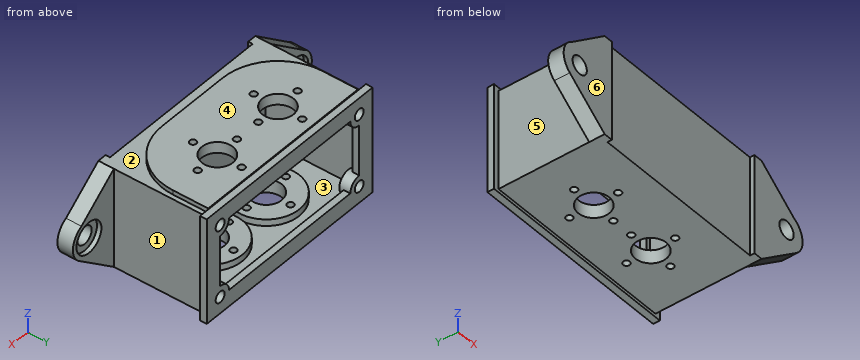
```python
from build123d import *

# Parameters (mm, degrees)
BOSS_EXTRUDE5_DEPTH  = 7
SKETCH10_W           = 88
SKETCH10_H           = 45
SKETCH10_W_2         = 82
SKETCH10_H_2         = 39
BOSS_EXTRUDE6_DEPTH  = 41
SKETCH11_W           = 93
SKETCH11_H           = 48
SKETCH11_W_2         = 78
SKETCH11_H_2         = 33
BOSS_EXTRUDE7_DEPTH  = 3
SKETCH12_R           = 5
BOSS_EXTRUDE8_DEPTH  = 5
SKETCH13_R           = 2.5
CUT_EXTRUDE1_DEPTH   = 5
SKETCH14_R           = 15
BOSS_EXTRUDE9_DEPTH  = 3
SKETCH16_R           = 7
CUT_EXTRUDE2_DEPTH   = 22
SKETCH17_R           = 1.5
CUT_EXTRUDE3_DEPTH   = 22
SKETCH18_W           = 80
SKETCH18_H           = 2
CUT_EXTRUDE4_DEPTH   = 92
BOSS_EXTRUDE11_DEPTH = 2
SKETCH20_R           = 7
CUT_EXTRUDE5_DEPTH   = 14
SKETCH21_R           = 1.5
CUT_EXTRUDE6_DEPTH   = 14
SKETCH22_R           = 4
CUT_EXTRUDE8_DEPTH   = 14
SKETCH23_R           = 7
CUT_EXTRUDE9_DEPTH   = 2


with BuildPart() as part:
    # Sketch9 → Boss-Extrude5 (new body)
    with BuildSketch(Plane(origin=(0, 0, 0), x_dir=(1, 0, 0), z_dir=(0, 1, 0))):
        with BuildLine():
            Line((-44, 22.5), (44, 22.5))
            Line((44, 22.5), (63.572502172, 7.067334685))
            ThreePointArc((63.572502172, 7.067334685), (66.961735718, -0.829031319), (62.181462037, -7.969653395))
            Line((62.181462037, -7.969653395), (44, -22.5))
            Line((44, -22.5), (-44, -22.5))
            Line((-44, -22.5), (-62.181462037, -7.969653395))
            ThreePointArc((-62.181462037, -7.969653395), (-66.961735718, -0.829031319), (-63.572502172, 7.067334685))
            Line((-63.572502172, 7.067334685), (-44, 22.5))
        make_face()
    extrude(amount=BOSS_EXTRUDE5_DEPTH)

    # Sketch10 → Boss-Extrude6 (add)
    with BuildSketch(Plane(origin=(0, 7, 0), x_dir=(1, 0, 0), z_dir=(0, 1, 0))):
        Rectangle(SKETCH10_W, SKETCH10_H)
        Rectangle(SKETCH10_W_2, SKETCH10_H_2, mode=Mode.SUBTRACT)
    extrude(amount=BOSS_EXTRUDE6_DEPTH)

    # Sketch11 → Boss-Extrude7 (add)
    with BuildSketch(Plane(origin=(0, 48, 0), x_dir=(1, 0, 0), z_dir=(0, 1, 0))):
        Rectangle(SKETCH11_W, SKETCH11_H)
        Rectangle(SKETCH11_W_2, SKETCH11_H_2, mode=Mode.SUBTRACT)
    extrude(amount=BOSS_EXTRUDE7_DEPTH)

    # Sketch12 → Boss-Extrude8 (add)
    with BuildSketch(Plane(origin=(0, 51, 0), x_dir=(1, 0, 0), z_dir=(0, 1, 0))):
        with Locations((39, 16.5)):
            Circle(SKETCH12_R)
        with Locations((39, -16.5)):
            Circle(SKETCH12_R)
        with Locations((-39, -16.5)):
            Circle(SKETCH12_R)
        with Locations((-39, 16.5)):
            Circle(SKETCH12_R)
    extrude(amount=-BOSS_EXTRUDE8_DEPTH)

    # Sketch13 → Cut-Extrude1 (cut)
    with BuildSketch(Plane(origin=(0, 51, 0), x_dir=(1, 0, 0), z_dir=(0, 1, 0))):
        with Locations(Location((39, 16.5, 0), (0, 0, 270))):
            Circle(SKETCH13_R)
        with Locations(Location((39, -16.5, 0), (0, 0, 323.130102354))):
            Circle(SKETCH13_R)
        with Locations(Location((-39, 16.5, 0), (0, 0, 216.869897646))):
            Circle(SKETCH13_R)
        with Locations(Location((-39, -16.5, 0), (0, 0, 270))):
            Circle(SKETCH13_R)
    extrude(amount=-CUT_EXTRUDE1_DEPTH, mode=Mode.SUBTRACT)

    # Sketch14 → Boss-Extrude9 (add)
    with BuildSketch(Plane.XY.offset(-19.5)):
        with Locations((16, 27.5)):
            Circle(SKETCH14_R)
        with Locations(Location((-16, 27.5, 0), (0, 0, 180))):
            Circle(SKETCH14_R)
    extrude(amount=BOSS_EXTRUDE9_DEPTH)

    # Sketch16 → Cut-Extrude2 (cut)
    with BuildSketch(Plane.XY.offset(-16.5)):
        with Locations((-16, 27.5)):
            Circle(SKETCH16_R)
        with Locations((16, 27.5)):
            Circle(SKETCH16_R)
    extrude(amount=-CUT_EXTRUDE2_DEPTH, mode=Mode.SUBTRACT)

    # Sketch17 → Cut-Extrude3 (cut)
    with BuildSketch(Plane.XY.offset(-16.5)):
        with Locations((16, 38.5)):
            Circle(SKETCH17_R)
        with Locations((27, 27.5)):
            Circle(SKETCH17_R)
        with Locations((16, 16.5)):
            Circle(SKETCH17_R)
        with Locations((5, 27.5)):
            Circle(SKETCH17_R)
        with Locations((-5, 27.5)):
            Circle(SKETCH17_R)
        with Locations((-16, 16.5)):
            Circle(SKETCH17_R)
        with Locations((-27, 27.5)):
            Circle(SKETCH17_R)
        with Locations((-16, 38.5)):
            Circle(SKETCH17_R)
    extrude(amount=-CUT_EXTRUDE3_DEPTH, mode=Mode.SUBTRACT)

    # Sketch18 → Cut-Extrude4 (cut)
    with BuildSketch(Plane.XY.offset(22.5)):
        with Locations((0, 1)):
            Rectangle(SKETCH18_W, SKETCH18_H)
    extrude(amount=-CUT_EXTRUDE4_DEPTH, mode=Mode.SUBTRACT)

    # Sketch19 → Boss-Extrude11 (add)
    with BuildSketch(Plane.XY.offset(22.5)):
        with BuildLine():
            Line((-42, 48), (42, 48))
            Line((42, 48), (42, 32))
            ThreePointArc((42, 32), (34.67766953, 14.32233047), (17, 7))
            Line((17, 7), (-17, 7))
            ThreePointArc((-17, 7), (-34.67766953, 14.32233047), (-42, 32))
            Line((-42, 32), (-42, 48))
        make_face()
    extrude(amount=BOSS_EXTRUDE11_DEPTH)

    # Sketch20 → Cut-Extrude5 (cut)
    with BuildSketch(Plane.XY.offset(24.5)):
        with Locations((-17, 32)):
            Circle(SKETCH20_R)
        with Locations(Location((17, 32, 0), (0, 0, 180))):
            Circle(SKETCH20_R)
    extrude(amount=-CUT_EXTRUDE5_DEPTH, mode=Mode.SUBTRACT)

    # Sketch21 → Cut-Extrude6 (cut)
    with BuildSketch(Plane.XY.offset(24.5)):
        with Locations((-17, 43)):
            Circle(SKETCH21_R)
        with Locations((-6, 32)):
            Circle(SKETCH21_R)
        with Locations((-17, 21)):
            Circle(SKETCH21_R)
        with Locations((-28, 32)):
            Circle(SKETCH21_R)
        with Locations(Location((17, 21, 0), (0, 0, 180))):
            Circle(SKETCH21_R)
        with Locations(Location((28, 32, 0), (0, 0, 180))):
            Circle(SKETCH21_R)
        with Locations(Location((17, 43, 0), (0, 0, 180))):
            Circle(SKETCH21_R)
        with Locations(Location((6, 32, 0), (0, 0, 180))):
            Circle(SKETCH21_R)
    extrude(amount=-CUT_EXTRUDE6_DEPTH, mode=Mode.SUBTRACT)

    # Sketch22 → Cut-Extrude8 (cut)
    with BuildSketch(Plane(origin=(0, 7, 0), x_dir=(1, 0, 0), z_dir=(0, 1, 0))):
        with Locations(Location((-58, 0, 0), (0, 0, 270))):
            Circle(SKETCH22_R)
        with Locations(Location((58, 0, 0), (0, 0, 90))):
            Circle(SKETCH22_R)
    extrude(amount=-CUT_EXTRUDE8_DEPTH, mode=Mode.SUBTRACT)

    # Sketch23 → Cut-Extrude9 (cut)
    with BuildSketch(Plane(origin=(0, 7, 0), x_dir=(1, 0, 0), z_dir=(0, 1, 0))):
        with Locations(Location((-58, 0, 0), (0, 0, 270))):
            Circle(SKETCH23_R)
        with Locations(Location((58, 0, 0), (0, 0, 90))):
            Circle(SKETCH23_R)
    extrude(amount=-CUT_EXTRUDE9_DEPTH, mode=Mode.SUBTRACT)


solid = part.part
```
For this review, take the finished solid that the model builds, in its own axes (mm). Face numbers are marked on the shaded views. A direction names the side the tool comes from. Round coordinates to 2 decimals unless told otherwise and drop trailing zeros. Order: outer loops, then holes, each group sorted by start corner. A loop starts at its lowest first (then second) coordinate and runs counter-clockwise, first axis right, second up.
Q1. We need section C-C, the plane y = 8.5. Give the boundary of the cut face in (x, z).
Findings below:
outline: (-44, -22.5) - (44, -22.5) - (44, 22.5) - (25.53, 22.5) - (25.53, 24.5) - (-25.53, 24.5) - (-25.53, 22.5) - (-44, 22.5) - close; hole (-41, -19.5) - (41, -19.5) - (41, 19.5) - (-41, 19.5) - close
Q2. Insertion check: P1, Ø3, axis at x = -39, z = 16.5, coming from the -Y side; P2, Ø2.5, axis at y = 50, z = 0, coming from the -X side; P3, Ø8, axis at x = 3.5, y = 14.5, coming from the -Z side; P4, Ø2, axis at x = -12, z = 2, coming from the -Y side. Each pin has a flat end and moves straight along its axis. Give the tip position at first contact, or say it passes through.
Findings below:
P1: stops at y = 0
P2: stops at x = -46.5
P3: stops at z = -22.5
P4: stops at y = 2
Q3. Wall thickness on line 1 (Z direction, x = 4.5, y = 9); line 2 (X direction, y = 47.65, z = -16.5); line 3 (Y direction, x = 6, z = 22.6): over which ranges is each line inside the solid? List them lowest first.
Findings below:
line 1: z = -22.5 to -19.5, 19.5 to 24.5
line 2: x = -44 to -41.5, -36.5 to -34, 34 to 36.5, 41.5 to 44
line 3: y = 7 to 30.5, 33.5 to 51
Q4. We need section B-B, the plane z = -21. State how many separate pieces and enclosed holes the cut face has, plus the area to 3 significant figures.
Findings below:
separate pieces: 1
enclosed holes: 10
area: 4,010 mm2
Q5. We need section D-D, the plane z = 9.5. Give the boundary of the cut face in (x, y).
Findings below:
outline: (-60.27, 0) - (-40, 0) - (-40, 2) - (40, 2) - (40, 0) - (60.27, 0) - (60.27, 7) - (44, 7) - (44, 48) - (46.5, 48) - (46.5, 51) - (39, 51) - (39, 48) - (41, 48) - (41, 7) - (-41, 7) - (-41, 48) - (-39, 48) - (-39, 51) - (-46.5, 51) - (-46.5, 48) - (-44, 48) - (-44, 7) - (-60.27, 7) - close
Q6. We need section A-A, the plane x = -58. Give the boundary of the cut face in (y, z).
Findings below:
outline: (0, -11.46) - (7, -11.46) - (7, -7) - (5, -7) - (5, -4) - (0, -4) - close; (0, 4) - (5, 4) - (5, 7) - (7, 7) - (7, 11.31) - (0, 11.31) - close
Q7. Mouldability with a two-part tool opening along Y and no side actions: class the marked faces 4, 5 and 6 as pulls with the +Y half, pulls with the -Y half, needs draft (parallel to the pull), parting line crosses it, or undercut.
Findings below:
face 4: needs draft
face 5: undercut
face 6: pulls with the -Y half
Q8. Machinability: for the marked faces 1, 2 and 3, which of the approach directions +Z, -Z, +X, -X, +Y, -Y give a long, thin tool a straight path to every point of the face, cutting with its end or side? Answer none if there is none.
Findings below:
face 1: +Z, -Z, +X
face 2: +Z, -Y
face 3: none
